from build123d import *

# Parameters (mm, degrees)
F1_DEPTH = 80
F2_R     = 2
F3_DEPTH = 25
F4_R     = 2.5
F5_DEPTH = 22
F4_R_2   = 3.1
F6_DEPTH = 5


# Not quite as in the source:
# - a feature names something its author has since deleted; it is built from what else it names


with BuildPart() as f1:
    # F0 (on Front) → F1 (new body)
    with BuildSketch(Plane.XZ):
        Polygon((-110, -25), (110, -25), (110, -15), (-90, -15), (-90, 25), (-110, 25), align=None)
    extrude(amount=F1_DEPTH)

    # F2 (on face) → F3 (cut)
    with BuildSketch(Plane.XY.offset(-15)):
        with Locations((-80, -40)):
            Circle(F2_R)
        with Locations((-50, -40)):
            Circle(F2_R)
        with Locations((-20, -40)):
            Circle(F2_R)
        with Locations((10, -40)):
            Circle(F2_R)
        with Locations((40, -40)):
            Circle(F2_R)
        with Locations((70, -40)):
            Circle(F2_R)
        with Locations((100, -40)):
            Circle(F2_R)
    extrude(amount=-F3_DEPTH, mode=Mode.SUBTRACT)

    # F4 (on face) → F5 (cut)
    with BuildSketch(Plane.YZ.offset(-90)):
        with Locations((-50, 12)):
            Circle(F4_R)
        with Locations((-30, 12)):
            Circle(F4_R)
    extrude(amount=-F5_DEPTH, mode=Mode.SUBTRACT)

    # F4 (on face) → F6 (cut)
    with BuildSketch(Plane.YZ.offset(-90)):
        with Locations((-40, 12)):
            Circle(F4_R_2)
    extrude(amount=-F6_DEPTH, mode=Mode.SUBTRACT)


solid = f1.part
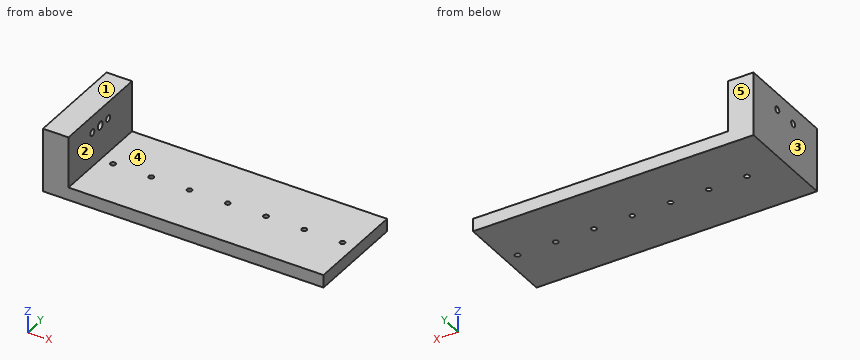
Input: part model. Units: mm. Frame: model coordinates. Face numbers are marked on the shaded views. A direction names the side the tool comes from. Coordinates: 2 decimals unless noted, no trailing zeros. Loops run counter-clockwise (first coordinate to the right, second up) from the corner with the lowest first, then second, coordinate; pieces in that order, holes last.
(1) Pull-direction query (X, two-part tool) for the marked faces 1, 2 and 3; classes: released by +X, released by -X, zero draft, split by the parting line, or undercut.
(2) Section B-B on y = -30. Return the cut outline in (x, z), then the cut area to 3 significant figures.
(3) Set-up query: the marked faces 4 and 5. Return all of +Z, -Z, +X, -X, +Y, -Y with unobstructed straight access to the full face (end or side cutting, diameter ignored); none if empty.
(4) Section C-C on z = 12. Return the cut outline in (x, y).
(5) Section A-A on x = 70. Return the cut outline in (y, z), then the cut area to 3 significant figures.
(6) Material intervals for probe 1 along Y at (x, z) = (-20, -17.5); probe 2 along Z at (x, y) = (-100, -30); probe 3 along Z at (x, y) = (-35, -21.5), sorted ascending.
(7) First-contact query: pin 1 Ø2.5 at (x, y) = (-50, -40) entering from +Z; pin 2 Ø6 at (x, y) = (-33.5, -58) entering from +Z; pin 3 Ø5 at (y, z) = (-40, 12) entering from +X; pin 4 Ø5 at (y, z) = (-40, 11) entering from +X. Flat tips, straight axial feed; report the tip coordinate or a pass-through.
(8) Section D-D on z = 21. Return the cut outline in (x, y), then the cut area to 3 significant figures.
Data:
1. face 1: zero draft
1. face 2: released by +X
1. face 3: released by -X
2. outline: (-110, -25) - (110, -25) - (110, -15) - (-90, -15) - (-90, 9.5) - (-110, 9.5) - close; (-110, 14.5) - (-90, 14.5) - (-90, 25) - (-110, 25) - close
2. area: 2,900 mm2
3. face 4: +Z, +X, +Y, -Y
3. face 5: +Z, -Z, +X, -X, +Y
4. outline: (-110, -80) - (-90, -80) - (-90, -52.5) - (-110, -52.5) - close; (-110, -47.5) - (-90, -47.5) - (-90, -43.1) - (-95, -43.1) - (-95, -36.9) - (-90, -36.9) - (-90, -32.5) - (-110, -32.5) - close; (-110, -27.5) - (-90, -27.5) - (-90, 0) - (-110, 0) - close
5. outline: (-80, -25) - (-42, -25) - (-42, -15) - (-80, -15) - close; (-38, -25) - (0, -25) - (0, -15) - (-38, -15) - close
5. area: 760 mm2
6. probe 1: y = -80 to -42, -38 to 0
6. probe 2: z = -25 to 9.5, 14.5 to 25
6. probe 3: z = -25 to -15
7. pin 1: passes through
7. pin 2: stops at z = -15
7. pin 3: stops at x = -95
7. pin 4: stops at x = -90
8. outline: (-110, -80) - (-90, -80) - (-90, 0) - (-110, 0) - close
8. area: 1,600 mm2
